Work out the finished part from the listing and answer in its coordinate system (mm). A direction names the side the tool comes from. Give positions to 0.01 mm unless a question says otherwise; leave off trailing zeros. Loops run counter-clockwise (first coordinate to the right, second up) from the corner with the lowest first, then second, coordinate; pieces in that order, holes last. Notation, with made-up numbers: (25.5, 71.25) - (82.5, 71.25) arc R12 cw to (82.5, 79.25) - close; hole circle Ø2 at (32, -20). An arc over 180 degrees is marked (long way). One line per question, with ' | ' between items.
from build123d import *

# Parameters (mm, degrees)
F0_R     = 7.25
F0_R_2   = 5.25
F1_DEPTH = 15
F2_R     = 15
F2_R_2   = 5.25
F3_DEPTH = 3
F4_R     = 15
F4_R_2   = 13
F5_DEPTH = 34.5


with BuildPart() as f1:
    # F0 (on Top) → F1 (new body)
    with BuildSketch(Plane.XY):
        Circle(F0_R)
        Circle(F0_R_2, mode=Mode.SUBTRACT)
    extrude(amount=-F1_DEPTH)

    # F2 (on face) → F3 (join)
    with BuildSketch(Plane.XY):
        with Locations((0.214589, 0)):
            Circle(F2_R)
        Circle(F2_R_2, mode=Mode.SUBTRACT)
    extrude(amount=F3_DEPTH)

    # F4 (on face) → F5 (join)
    with BuildSketch(Plane.XY.offset(3)):
        with Locations((0.214589, 0)):
            Circle(F4_R)
        with Locations((0.214589, 0)):
            Circle(F4_R_2, mode=Mode.SUBTRACT)
    extrude(amount=F5_DEPTH)


solid = f1.part
1. Find section B-B on x = 0. Write down the section's boundary in (y, z), then the cut area to 3 significant figures.
Evaluation:
outline: (-15, 0) - (-7.25, 0) - (-7.25, -15) - (-5.25, -15) - (-5.25, 3) - (-13, 3) - (-13, 37.5) - (-15, 37.5) - close; (5.25, -15) - (7.25, -15) - (7.25, 0) - (15, 0) - (15, 37.5) - (13, 37.5) - (13, 3) - (5.25, 3) - close | area: 257 mm2
2. Find section D-D on y = 9.5. Write down the section's boundary in (x, z).
Evaluation:
outline: (-11.39, 0) - (11.82, 0) - (11.82, 37.5) - (9.09, 37.5) - (9.09, 3) - (-8.66, 3) - (-8.66, 37.5) - (-11.39, 37.5) - close
3. Consider L1, parallel to Y at x = 0, z = -2; L2, parallel to Y at x = 0.5, z = 27; L3, parallel to Z at x = -1.5, y = -9.25. Determine where each line is inside the solid, lowest interval first.
Evaluation:
L1: -7.25 to -5.25, 5.25 to 7.25 | L2: -15 to -13, 13 to 15 | L3: 0 to 3
4. Which of the six approach directions +Z, -Z, +X, -X, +Y, -Y give full straight-line access (tool end or side, diameter ignored) to faces 4 (the flat face through (6, 0, 3)), 5 (the cylindrical face through (-14.77, 0.66, 18.49)), 6 (the flat face through (7, -3, 0))?
Evaluation:
face 4: +Z | face 5: +Z, -Z | face 6: -Z
5. Determine the mould class of faces 1 (the cylindrical face through (5, 1.6, -6.1)), 2 (the cylindrical face through (3.35, -6.43, -7.4)), 3 (the flat face through (-11, 7, 37.5)) for opening direction X: +X half, -X half, draft (parallel to the pull), parting line (faces both ways), or undercut.
Evaluation:
face 1: undercut | face 2: parting line | face 3: draft
6. Find section C-C on z = 26. Write down the section's boundary in (x, y), then the cut area to 3 significant figures.
Evaluation:
outline: circle Ø30 at (0.21, 0); hole circle Ø26 at (0.21, 0) | area: 176 mm2
7. Flat-ended cylindrical pins translate along their axes: pin 1 (6 mm diameter, centred on x = 8.5, z = 32, fed in from +Y); pin 2 (6 mm diameter, centred on y = -7, z = 3.5, fed in from +X); pin 3 (1 mm diameter, centred on y = -9.5, z = 1.5, fed in from +X). Find the tip coordinate at first contact, or state that the pin passes through.
Evaluation:
pin 1: y = 14.04 | pin 2: x = 14.67 | pin 3: x = 12.21
8. Find section A-A on y = 0. Write down the section's boundary in (x, z), then the cut area to 4 significant figures.
Evaluation:
outline: (-14.79, 0) - (-7.25, 0) - (-7.25, -15) - (-5.25, -15) - (-5.25, 3) - (-12.79, 3) - (-12.79, 37.5) - (-14.79, 37.5) - close; (5.25, -15) - (7.25, -15) - (7.25, 0) - (15.21, 0) - (15.21, 37.5) - (13.21, 37.5) - (13.21, 3) - (5.25, 3) - close | area: 256.5 mm2
